Here's how the part is built. I have some questions about the finished solid (model axes, mm). Face numbers are marked on the shaded views. A direction names the side the tool comes from. Coordinates: 2 decimals unless noted, no trailing zeros. Write each loop counter-clockwise with the first axis right and the second up, starting at its lowest first coordinate (ties: lowest second). Pieces come first, ordered by that corner, then holes. Notation, with made-up numbers: M -7.5,76 L 50.5,76 A22 cw 50.5,88 Z; hole C 45.5,-34 d6. An arc over 180 degrees is marked long. Use one line per item in the form item = value. Start each with the question number.
1. I want a section at B-B, the plane y = -15. List the corners of the cut face in (x, z) for me, plus the area to 3 significant figures.
2. Please list where these lines run through material, in increasing order: line 1 along Y through (x, z) = (5, 1.4); line 2 along Y through (x, z) = (0, 2.25); line 3 along X through (y, z) = (0, 2). Write a range as [from, to].
3. I want a section at C-C, the plane z = -1.5. List the corners of the cut face in (x, y) for me, plus the area to 3 significant figures.
4. I want a section at A-A, the plane x = 0. List the corners of the cut face in (y, z) for me.
5. Thinking about a two-plate mould opening in X: for the marked faces 1, 2 and 3, which applies, released by +X, released by -X, zero draft, split by the parting line, or undercut?
6. I want a section at D-D, the plane x = -21. List the corners of the cut face in (y, z) for me.
7. On a 3-axis mill with a long thin cutter (end or side, diameter ignored), from which of +Z, -Z, +X, -X, +Y, -Y can I reach the whole of each face in a straight line? I mean the marked faces 4 and 5. Say none if no direction works.
8. I'm going to push flat-ended pins straight in: pin 1 Ø0.8 at (y, z) = (10.5, 1) entering from +X; pin 2 Ø1.5 at (x, z) = (27, -4) entering from +Y; pin 3 Ø5 at (x, y) = (14.5, 18) entering from -Z. Where does each tip first touch, or does it pass through?
from build123d import *

# Parameters (mm, degrees)
SKETCH_1_R          = 28.3
SKETCH_1_R_2        = 20
EXTRUDE_1_DEPTH     = 2.5
EXTRUDE_START       = -2.5
SKETCH_2_R          = 1.6
EXTRUDE_2_DEPTH     = 2.5
EXTRUDE_START_2     = 5.2
EXTRUDE_3_DEPTH     = 5.2
EXTRUDE_START_3     = 1.5
EXTRUDE_4_DEPTH     = 1.5
CUT_EXTRUDE_START   = 10
CUT_EXTRUDE_1_DEPTH = 11.5
FILLET_1_R          = 3


with BuildPart() as part:
    # 草图1 → 凸台-拉伸1 (new body)
    with BuildSketch(Plane.XY):
        Circle(SKETCH_1_R)
        Circle(SKETCH_1_R_2, mode=Mode.SUBTRACT)
    extrude(amount=EXTRUDE_1_DEPTH)

    # 草图2 → 凸台-拉伸2 (add)
    with BuildSketch(Plane.XY.offset(2.5).offset(EXTRUDE_START)):
        with BuildLine():
            Line((-26.351833365, 10.318472674), (-12.5, 45.693979899))
            Line((-12.5, 45.693979899), (12.5, 45.693979899))
            Line((12.5, 45.693979899), (26.351833365, 10.318472674))
            ThreePointArc((26.351833365, 10.318472674), (0, 28.3), (-26.351833365, 10.318472674))
        make_face()
        with Locations((-5, 40.693979899)):
            Circle(SKETCH_2_R, mode=Mode.SUBTRACT)
        with Locations(Location((5, 40.693979899, 0), (0, 0, 180))):
            Circle(SKETCH_2_R, mode=Mode.SUBTRACT)
    extrude(amount=EXTRUDE_2_DEPTH)

    # 草图5 → 凸台-拉伸3 (add)
    with BuildSketch(Plane(origin=(0, 0, 0), x_dir=(-1, 0, 0), z_dir=(0, 0, -1)).offset(EXTRUDE_START_2)):
        with BuildLine():
            Line((-28.3, 0), (-26.3, 0))
            ThreePointArc((-26.3, 0), (0, -26.3), (26.3, 0))
            Line((26.3, 0), (28.3, 0))
            ThreePointArc((28.3, 0), (0, -28.3), (-28.3, 0))
        make_face()
    extrude(amount=-EXTRUDE_3_DEPTH)

    # 草图6 → 凸台-拉伸4 (add)
    with BuildSketch(Plane(origin=(0, 0, -5.2), x_dir=(-1, 0, 0), z_dir=(0, 0, -1)).offset(EXTRUDE_START_3)):
        with BuildLine():
            Line((-28.3, 0), (-25.3, 0))
            ThreePointArc((-25.3, 0), (0, -25.3), (25.3, 0))
            Line((25.3, 0), (28.3, 0))
            ThreePointArc((28.3, 0), (0, -28.3), (-28.3, 0))
        make_face()
    extrude(amount=-EXTRUDE_4_DEPTH)

    # 草图4 → 切除-拉伸1 (cut)
    with BuildSketch(Plane(origin=(0, 0, 0), x_dir=(-1, 0, 0), z_dir=(0, 0, -1)).offset(CUT_EXTRUDE_START)):
        with BuildLine():
            Line((-22.65, 0), (-22.65, 35.693979899))
            Line((-22.65, 35.693979899), (22.65, 35.693979899))
            Line((22.65, 35.693979899), (22.65, 0))
            ThreePointArc((22.65, 0), (0, -22.65), (-22.65, 0))
        make_face()
    extrude(amount=-CUT_EXTRUDE_1_DEPTH, mode=Mode.SUBTRACT)

    # 圆角1
    fillet_1_edges = [part.edges().sort_by_distance(p)[0] for p in [
        (-12.5, 45.693979899, 1.25),
        (12.5, 45.693979899, 1.25),
    ]]
    fillet(fillet_1_edges, radius=FILLET_1_R)


solid = part.part
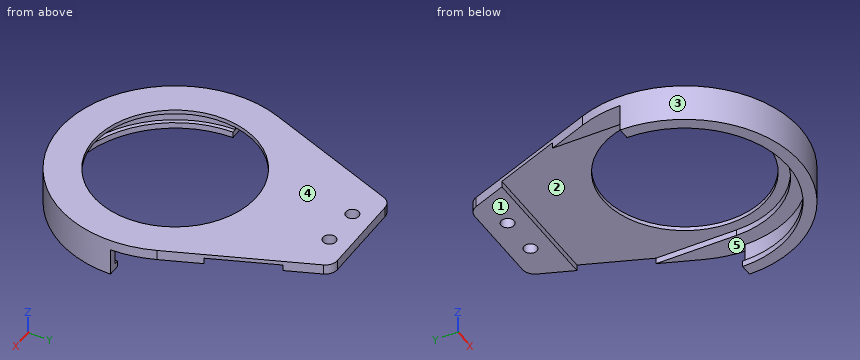
Answer list:
q1.outline = M -24,-6.7 L -20.37,-6.7 L -20.37,-5.2 L -21.6,-5.2 L -21.6,0 L -16.97,0 L -16.97,1.5 L -13.23,1.5 L -13.23,2.5 L -24,2.5 Z; M 13.23,1.5 L 16.97,1.5 L 16.97,0 L 21.6,0 L 21.6,-5.2 L 20.37,-5.2 L 20.37,-6.7 L 24,-6.7 L 24,2.5 L 13.23,2.5 Z
q1.area = 78.4 mm²
q2.line_1 = [-27.85, -22.09], [35.69, 39.09], [42.29, 45.69]
q2.line_2 = [-28.3, -20], [20, 45.69]
q2.line_3 = [-28.3, -20], [20, 28.3]
q3.outline = M -28.3,0 A28.3 ccw 28.3,0 L 26.3,0 A26.3 cw -26.3,0 Z
q3.area = 172 mm²
q4.outline = M -28.3,-6.7 L -25.3,-6.7 L -25.3,-5.2 L -26.3,-5.2 L -26.3,0 L -22.65,0 L -22.65,1.5 L -20,1.5 L -20,2.5 L -28.3,2.5 Z; M 20,1.5 L 35.69,1.5 L 35.69,0 L 45.69,0 L 45.69,2.5 L 20,2.5 Z
q5.face_1 = zero draft
q5.face_2 = undercut
q5.face_3 = split by the parting line
q6.outline = M -18.97,-6.7 L -14.11,-6.7 L -14.11,-5.2 L -15.83,-5.2 L -15.83,0 L -8.49,0 L -8.49,1.5 L 23.99,1.5 L 23.99,2.5 L -18.97,2.5 Z
q7.face_4 = +Z, +X, -X, +Y, -Y
q7.face_5 = +Y
q8.pin_1 = 26.44
q8.pin_2 = 0
q8.pin_3 = 1.5
